Source: CAD feature listing. Evaluate the final solid. Frame: model axes, mm. Face numbers are marked on the shaded views. A direction names the side the tool comes from. Coordinates: 2 decimals unless noted, no trailing zeros. Write each loop counter-clockwise with the first axis right and the second up, starting at its lowest first coordinate (ties: lowest second). Pieces come first, ordered by that corner, then holes. Notation, with made-up numbers: M 85.5,-26 L 139.5,-26 A18 cw 139.5,-20 Z; hole C 35.25,62 d10. An arc over 180 degrees is marked long. One line per item, written item: value. Start each with the question number.
Item 1: Pin query (flat end, axial travel): P1, Ø6, axis at x = -10.5, z = 112, coming from the +Y side; P2, Ø1, axis at x = -14, z = 61, coming from the -Y side; P3, Ø8, axis at y = -8.5, z = 97, coming from the +X side. Return the tip coordinate at first contact, or that it passes through.
Item 2: Ray query, L1, parallel to Z at x = 0, y = -16; L2, parallel to Y at x = 0, z = 34; L3, parallel to X at y = -1, z = 48. Return the intervals inside material, ascending. Write a range as from..to.
Item 3: Cut plane A-A, the plane y = 0. Output: boundary loops of the cut face in (x, z).
Item 4: Cut plane C-C, the plane z = 27.5. Output: boundary loops of the cut face in (x, y), then the cut area to 3 significant figures.
Item 5: Cut plane D-D, the plane z = 105. Output: boundary loops of the cut face in (x, y), then the cut area to 3 significant figures.
Item 6: Set-up query: the marked faces 1 and 2. Return all of +Z, -Z, +X, -X, +Y, -Y with unobstructed straight access to the full face (end or side cutting, diameter ignored); none if empty.
Item 7: Mould query, pull axis Z, two halves, no side actions, for the marked faces 3, 4 and 5. Classes: released by +Z, released by -Z, zero draft, split by the parting line, or undercut.
```python
from build123d import *

# Parameters (mm, degrees)
F0_R     = 35.2250481383
F1_DEPTH = 127
F2_SIZE2 = 50.8
F2_SIZE  = 12.7
F3_R     = 12.730483267
F4_DEPTH = 25.4


with BuildPart() as f1:
    # F0 (on Top) → F1 (new body)
    with BuildSketch(Plane.XY):
        Circle(F0_R)
    extrude(amount=F1_DEPTH)

    # F2
    f2_edges = [f1.edges().sort_by_distance(p)[0] for p in [
        (-35.225048, 0, 127),
    ]]
    f2_side = f1.faces().sort_by_distance((0, 0, 127))[0]
    chamfer(f2_edges, length=F2_SIZE, length2=F2_SIZE2, reference=f2_side)

    # F3 (on face) → F4 (join)
    with BuildSketch(Plane.XY.offset(127)):
        Circle(F3_R)
    extrude(amount=F4_DEPTH)


solid = f1.part
```
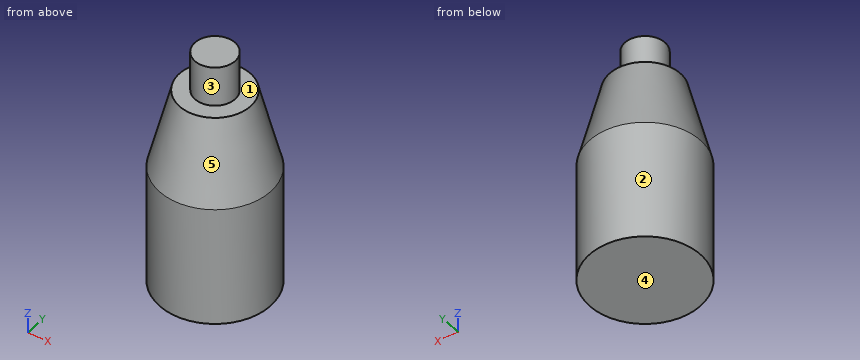
From the geometry:
1. P1: stops at y = 25.47
1. P2: stops at y = -32.54
1. P3: stops at x = 30.22
2. L1: z = 0..127
2. L2: y = -35.23..35.23
2. L3: x = -35.21..35.21
3. outline: M -35.23,0 L 35.23,0 L 35.23,76.2 L 22.53,127 L 12.73,127 L 12.73,152.4 L -12.73,152.4 L -12.73,127 L -22.53,127 L -35.23,76.2 Z
4. outline: C 0,0 d70.45
4. area: 3,900 mm²
5. outline: C 0,0 d56.05
5. area: 2,470 mm²
6. face 1: +Z
6. face 2: +Z, -Z
7. face 3: zero draft
7. face 4: released by -Z
7. face 5: released by +Z
